Check sheet for the modelled part. Datum: model origin and axes. Units: mm. Face numbers are marked on the shaded views. Give positions to 0.01 mm unless a question says otherwise; leave off trailing zeros. Order: outer loops, then holes, each group sorted by start corner. A loop starts at its lowest first (then second) coordinate and runs counter-clockwise, first axis right, second up. Notation, with made-up numbers: M -12,59 L 18,59 A19 ccw 18,67 Z; hole C 5,36 d5. An arc over 180 degrees is marked long. One line per question, with ' | ' between items. Start each with the question number.
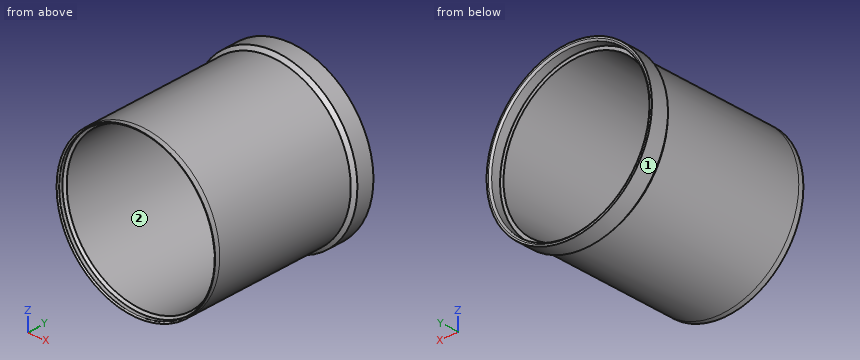
```python
from build123d import *

# Parameters (mm, degrees)
SKETCH1_R                = 36.8
SKETCH1_R_2              = 35.2
BOSS_EXTRUDE1_DEPTH      = 70
BOSS_EXTRUDE2_DEPTH      = 5
BOSS_EXTRUDE2_DEPTH_BACK = 5
SKETCH2_R                = 38.4
SKETCH2_R_2              = 36.8
CHAMFER1_SIZE            = 2
FILLET1_R                = 0.8
BOSS_EXTRUDE3_START      = 2.3
SKETCH3_R                = 36.8
SKETCH3_R_2              = 36.2
BOSS_EXTRUDE3_DEPTH      = 2.3
CHAMFER2_SIZE            = 1
FILLET2_R                = 0.6


# Some blends are built 0.0001 mm under size
with BuildPart() as part:
    # Sketch1 → Boss-Extrude1 (new body)
    with BuildSketch(Plane(origin=(0, 0, 0), x_dir=(1, 0, 0), z_dir=(0, 1, 0))):
        with Locations(Location((0, 0, 0), (0, 0, 270))):
            Circle(SKETCH1_R)
        with Locations(Location((0, 0, 0), (0, 0, 270))):
            Circle(SKETCH1_R_2, mode=Mode.SUBTRACT)
    extrude(amount=BOSS_EXTRUDE1_DEPTH)

    # Sketch2 → Boss-Extrude2 (add, two sides: drawn at the far end of the back side and taken through both)
    with BuildSketch(Plane(origin=(0, 70, 0), x_dir=(1, 0, 0), z_dir=(0, 1, 0)).offset(-BOSS_EXTRUDE2_DEPTH_BACK)):
        with Locations(Location((0, 0, 0), (0, 0, 270))):
            Circle(SKETCH2_R)
        with Locations(Location((0, 0, 0), (0, 0, 270))):
            Circle(SKETCH2_R_2, mode=Mode.SUBTRACT)
    extrude(amount=BOSS_EXTRUDE2_DEPTH + BOSS_EXTRUDE2_DEPTH_BACK)

    # Chamfer1
    # the kernel refuses this chamfer: 2 mm, written as the material it takes off along each edge
    with BuildSketch(Plane(origin=(0, 65, 0), x_dir=(0, 0, 1), z_dir=(-1, 0, 0))) as chamfer1_piece_1_section:
        Polygon((38.4 - CHAMFER1_SIZE, 0), (38.4, CHAMFER1_SIZE), (38.4, 0), align=None)
    chamfer1_piece_1 = revolve(axis=Axis((0, 65, 0), (0, 1, 0)), mode=Mode.PRIVATE)
    chamfer1_piece_1 = chamfer1_piece_1 - Plane(origin=(0, 66.172330508, 0), x_dir=(0, 0, 1), z_dir=(0, -1, 0)) * Cylinder(36.8, 154, mode=Mode.PRIVATE)
    add(chamfer1_piece_1, mode=Mode.SUBTRACT)

    # Fillet1
    fillet1_edges = [part.edges().sort_by_distance(p)[0] for p in [
        (0, 75, -36.8),
    ]]
    fillet(fillet1_edges, radius=FILLET1_R)

    # Sketch3 → Boss-Extrude3 (add)
    with BuildSketch(Plane.XZ.offset(BOSS_EXTRUDE3_START)):
        with Locations(Location((0, 0, 0), (0, 0, 270))):
            Circle(SKETCH3_R)
        with Locations(Location((0, 0, 0), (0, 0, 270))):
            Circle(SKETCH3_R_2, mode=Mode.SUBTRACT)
    extrude(amount=-BOSS_EXTRUDE3_DEPTH)

    # Chamfer2
    chamfer2_edges = [part.edges().sort_by_distance(p)[0] for p in [
        (0, 0, -35.2),
    ]]
    chamfer(chamfer2_edges, length=CHAMFER2_SIZE - 0.0001)  # a hair under: the kernel refuses the full size

    # Fillet2
    fillet2_edges = [part.edges().sort_by_distance(p)[0] for p in [
        (0, -2.3, 36.2),
    ]]
    fillet(fillet2_edges, radius=FILLET2_R - 0.0001)  # a hair under: the kernel refuses the full size


solid = part.part
```
Item 1: Scan lines: probe 1 along X at (y, z) = (22, 0); probe 2 along Z at (x, y) = (30, 24); probe 3 along Z at (x, y) = (-5, 42). Record each from-to range of solid material in increasing order. Write a range as [from, to].
Item 2: Go/stop test with flat-tipped pins: P1, Ø1, axis at y = 59, z = -2.5, coming from the +X side; P2, Ø3, axis at x = 9, y = 44.5, coming from the -Z side; P3, Ø1.5, axis at x = 19, y = 21, coming from the -Z side. Record where each tip stops, or that it passes through.
Item 3: Draft check along Z on the marked faces 1 and 2. Enter one of: released by +Z, released by -Z, zero draft, split by the parting line, or undercut.
Item 4: Section check C-C, the plane y = 47. Record the cut outline in (x, z).
Reported:
1) probe 1: x = [-36.8, -35.2], [35.2, 36.8] | probe 2: z = [-21.31, -18.41], [18.41, 21.31] | probe 3: z = [-36.46, -34.84], [34.84, 36.46]
2) P1: stops at x = 36.75 | P2: stops at z = -36.03 | P3: stops at z = -31.96
3) face 1: split by the parting line | face 2: undercut
4) outline: C 0,0 d73.6; hole C 0,0 d70.4
